Source: three-view drawing plus pictorial views. Frame: mm from the lowest corner of the part. A direction names the side the tool comes from. Give positions to 0.01 mm unless a question says otherwise; leave off trailing zeros. Write each loop counter-clockwise with the first axis right and the second up, starting at its lowest first coordinate (ties: lowest second). Pieces come first, ordered by that corner, then holes.
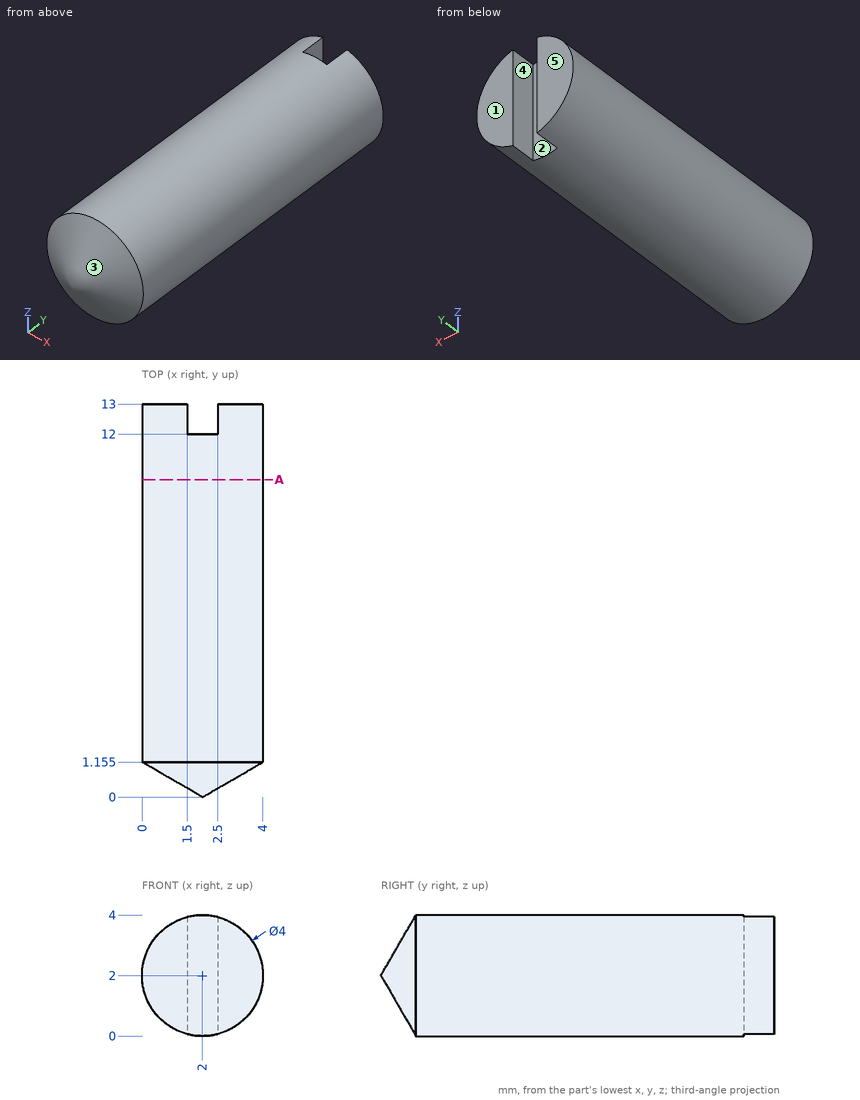
Q1. Pin query (flat end, axial travel): P1, Ø2, axis at y = 3, z = 0.5, coming from the +X side; P2, Ø0.5, axis at x = 2, z = 2.5, coming from the +Y side; P3, Ø0.8, axis at y = 12.5, z = 2.5, coming from the +X side. Return the tip coordinate at first contact, or that it passes through.
Filled sheet:
P1: stops at x = 3.94
P2: stops at y = 12
P3: stops at x = 4
Q2. Section A-A on y = 10.5. Output: boundary loops of the cut face in (x, z), plus the area to 3 significant figures.
Filled sheet:
outline: circle Ø4 at (2, 2)
area: 12.6 mm2
Q3. Pull-direction query (X, two-part tool) for the marked faces 1, 2 and 3; classes: released by +X, released by -X, zero draft, split by the parting line, or undercut.
Filled sheet:
face 1: zero draft
face 2: undercut
face 3: split by the parting line
Q4. Access query for the marked faces 4 and 5. Directions: +Z, -Z, +X, -X, +Y, -Y. A direction counts if a zero-diameter tool reaches every point of the face in a straight line with its end or side. Return the directions, or none.
Filled sheet:
face 4: +Z, -Z, +Y
face 5: +Z, -Z, +X, -X, +Y
Q5. Ray query, line 1 along Y through (x, z) = (3, 1); line 2 along Z through (x, y) = (0.5, 3.5); line 3 along Z through (x, y) = (0.85, 2) (1 decimal). Return the intervals inside material, ascending.
Filled sheet:
line 1: y = 0.82 to 13
line 2: z = 0.68 to 3.32
line 3: z = 0.4 to 3.6
